from build123d import *

# Parameters (mm, degrees)
BASE_FLANGE1_START             = -11.5
BASE_FLANGE1_DEPTH             = 23
EDGE_FLANGE1_STRIP_W           = 7.0732
EDGE_FLANGE1_STRIP_H           = 1.4
EDGE_FLANGE1_STRIP_CUT_DEPTH   = 39.1268
EDGE_FLANGE1_STRIP_2_W         = 7.0732
EDGE_FLANGE1_STRIP_2_H         = 1.4
EDGE_FLANGE1_STRIP_CUT_2_DEPTH = 39.1268
EDGE_FLANGE1_DEPTH             = 39.1268
EDGE_FLANGE1_BEND_DEPTH        = 39.1268
FILLET1_RADIUS                 = 11.5
FILLET1_LENGTH                 = 1.4
CUT_EXTRUDE1_REACH             = 58.319
SKETCH12_R                     = 4.05
SKETCH12_R_2                   = 0.9
SKETCH13_R                     = 4.075
SKETCH13_R_2                   = 0.9
CUT_EXTRUDE2_DEPTH             = 42.942102952
FILLET2_R                      = 0.5
CUT_EXTRUDE3_REACH             = 58.319
SKETCH14_R                     = 4.05
SKETCH14_R_2                   = 0.9


# Read off the part's stored shape, not the designer's step: Base-Flange1
# Sheet-metal steps are written as plain solids
with BuildPart() as part:
    # Base-Flange1 outline → Base-Flange1 (new body)
    with BuildSketch(Plane(origin=(0, 0, 0), x_dir=(0, 0, -1), z_dir=(1, 0, 0)).offset(BASE_FLANGE1_START)):
        with BuildLine():
            Line((21.7, 2.1366), (21.7, 34))
            Line((21.7, 34), (20.3, 34))
            Line((20.3, 34), (20.3, 2.1366))
            ThreePointArc((20.3, 2.1366), (20.084254855, 1.615745145), (19.5634, 1.4))
            Line((19.5634, 1.4), (-19.5634, 1.4))
            ThreePointArc((-19.5634, 1.4), (-20.084254855, 1.615745145), (-20.3, 2.1366))
            Line((-20.3, 2.1366), (-20.3, 34))
            Line((-20.3, 34), (-21.7, 34))
            Line((-21.7, 34), (-21.7, 2.1366))
            ThreePointArc((-21.7, 2.1366), (-21.074204349, 0.625795651), (-19.5634, 0))
            Line((-19.5634, 0), (19.5634, 0))
            ThreePointArc((19.5634, 0), (21.074204349, 0.625795651), (21.7, 2.1366))
        make_face()
    extrude(amount=BASE_FLANGE1_DEPTH)

    # Edge-Flange1 strip (across the edge) → Edge-Flange1 strip cut (cut)
    with BuildSketch(Plane(origin=(11.5, 1.4, 19.5634), x_dir=(-1, 0, 0), z_dir=(0, 0, -1))):
        with Locations((-1.4, -0.7)):
            Rectangle(EDGE_FLANGE1_STRIP_W, EDGE_FLANGE1_STRIP_H)
    extrude(amount=EDGE_FLANGE1_STRIP_CUT_DEPTH, mode=Mode.SUBTRACT)

    # Edge-Flange1 strip 2 (across the edge) → Edge-Flange1 strip cut 2 (cut)
    with BuildSketch(Plane(origin=(-11.5, 1.4, -19.5634), x_dir=(1, 0, 0), z_dir=(0, 0, 1))):
        with Locations((-1.4, -0.7)):
            Rectangle(EDGE_FLANGE1_STRIP_2_W, EDGE_FLANGE1_STRIP_2_H)
    extrude(amount=EDGE_FLANGE1_STRIP_CUT_2_DEPTH, mode=Mode.SUBTRACT)

    # Edge-Flange1 section (across the edge) → Edge-Flange1 (add)
    with BuildSketch(Plane(origin=(11.5, 1.4, 19.5634), x_dir=(-1, 0, 0), z_dir=(0, 0, -1))):
        with BuildLine():
            Line((0, 0.7366), (0, 3.6))
            Line((0, 3.6), (1.4, 3.6))
            Line((1.4, 3.6), (1.4, 0.7366))
            ThreePointArc((1.4, 0.7366), (1.615745145, 0.215745145), (2.1366, 0))
            Line((2.1366, 0), (2.1366, -1.4))
            ThreePointArc((2.1366, -1.4), (0.625795651, -0.774204349), (0, 0.7366))
        make_face()
    extrude(amount=EDGE_FLANGE1_DEPTH)

    # Edge-Flange1 section 2 (across the edge) → Edge-Flange1 bend (add)
    with BuildSketch(Plane(origin=(-11.5, 1.4, -19.5634), x_dir=(1, 0, 0), z_dir=(0, 0, 1))):
        with BuildLine():
            Line((0, 0.7366), (0, 3.6))
            Line((0, 3.6), (1.4, 3.6))
            Line((1.4, 3.6), (1.4, 0.7366))
            ThreePointArc((1.4, 0.7366), (1.615745145, 0.215745145), (2.1366, 0))
            Line((2.1366, 0), (2.1366, -1.4))
            ThreePointArc((2.1366, -1.4), (0.625795651, -0.774204349), (0, 0.7366))
        make_face()
    extrude(amount=EDGE_FLANGE1_BEND_DEPTH)

    # Fillet1: full round fillet: the end face becomes a half cylinder, R = half its width
    fillet1_face = Plane((0, 34, 21), x_dir=(0, 0, 1), z_dir=(0, 1, 0))  # on the end face: x along it, z out of the body
    fillet1_slab = fillet1_face.offset(-FILLET1_RADIUS / 2) * Box(FILLET1_LENGTH, 2 * FILLET1_RADIUS, FILLET1_RADIUS, mode=Mode.PRIVATE)  # the body's end, R deep
    fillet1_round = Plane((0, 22.5, 21), x_dir=(0, 1, 0), z_dir=(0, 0, 1)) * Cylinder(FILLET1_RADIUS, FILLET1_LENGTH, mode=Mode.PRIVATE)  # its axis R under the face
    add(fillet1_slab - fillet1_round, mode=Mode.SUBTRACT)

    # Sketch12 → Cut-Extrude1 (cut, up to next)
    with BuildSketch(Plane.XY.offset(21.7), mode=Mode.PRIVATE) as cut_extrude1_sk1:
        with Locations((0, 22.5)):
            Circle(SKETCH12_R)
    cut_extrude1_tool1 = extrude(cut_extrude1_sk1.sketch, amount=-CUT_EXTRUDE1_REACH, mode=Mode.PRIVATE) & part.part
    # Sketch12 → Cut-Extrude1 (cut, up to next)
    with BuildSketch(Plane.XY.offset(21.7), mode=Mode.PRIVATE) as cut_extrude1_sk2:
        with Locations((0, 29.5)):
            Circle(SKETCH12_R_2)
    cut_extrude1_tool2 = extrude(cut_extrude1_sk2.sketch, amount=-CUT_EXTRUDE1_REACH, mode=Mode.PRIVATE) & part.part
    # Sketch12 → Cut-Extrude1 (cut, up to next)
    with BuildSketch(Plane.XY.offset(21.7), mode=Mode.PRIVATE) as cut_extrude1_sk3:
        with Locations((7, 22.5)):
            Circle(SKETCH12_R_2)
    cut_extrude1_tool3 = extrude(cut_extrude1_sk3.sketch, amount=-CUT_EXTRUDE1_REACH, mode=Mode.PRIVATE) & part.part
    # Sketch12 → Cut-Extrude1 (cut, up to next)
    with BuildSketch(Plane.XY.offset(21.7), mode=Mode.PRIVATE) as cut_extrude1_sk4:
        with Locations((0, 15.5)):
            Circle(SKETCH12_R_2)
    cut_extrude1_tool4 = extrude(cut_extrude1_sk4.sketch, amount=-CUT_EXTRUDE1_REACH, mode=Mode.PRIVATE) & part.part
    # Sketch12 → Cut-Extrude1 (cut, up to next)
    with BuildSketch(Plane.XY.offset(21.7), mode=Mode.PRIVATE) as cut_extrude1_sk5:
        with Locations((-7, 22.5)):
            Circle(SKETCH12_R_2)
    cut_extrude1_tool5 = extrude(cut_extrude1_sk5.sketch, amount=-CUT_EXTRUDE1_REACH, mode=Mode.PRIVATE) & part.part
    add(cut_extrude1_tool1.solids().sort_by_distance((0, 22.5, 21.7))[0], mode=Mode.SUBTRACT)
    add(cut_extrude1_tool2.solids().sort_by_distance((0, 29.5, 21.7))[0], mode=Mode.SUBTRACT)
    add(cut_extrude1_tool3.solids().sort_by_distance((7, 22.5, 21.7))[0], mode=Mode.SUBTRACT)
    add(cut_extrude1_tool4.solids().sort_by_distance((0, 15.5, 21.7))[0], mode=Mode.SUBTRACT)
    add(cut_extrude1_tool5.solids().sort_by_distance((-7, 22.5, 21.7))[0], mode=Mode.SUBTRACT)

    # Sketch13 → Cut-Extrude2 (cut, through all)
    with BuildSketch(Plane(origin=(0, 0, 0), x_dir=(1, 0, 0), z_dir=(0, 1, 0))):
        with Locations(Location((0, 0, 0), (0, 0, 270))):
            Circle(SKETCH13_R)
        with Locations(Location((-4.87903679, 4.87903679, 0), (0, 0, 270))):
            Circle(SKETCH13_R_2)
        with Locations(Location((4.87903679, 4.87903679, 0), (0, 0, 270))):
            Circle(SKETCH13_R_2)
        with Locations(Location((4.87903679, -4.87903679, 0), (0, 0, 270))):
            Circle(SKETCH13_R_2)
        with Locations(Location((-4.87903679, -4.87903679, 0), (0, 0, 270))):
            Circle(SKETCH13_R_2)
        with Locations(Location((0, 13.35, 0), (0, 0, 270))):
            Circle(SKETCH13_R_2)
        with Locations(Location((0, -13.35, 0), (0, 0, 90))):
            Circle(SKETCH13_R_2)
    extrude(amount=CUT_EXTRUDE2_DEPTH, mode=Mode.SUBTRACT)

    # Fillet2
    fillet2_edges = [part.edges().sort_by_distance(p)[0] for p in [
        (-11.5, 34, -21),
        (11.5, 34, -21),
    ]]
    fillet(fillet2_edges, radius=FILLET2_R)

    # Sketch14 → Cut-Extrude3 (cut, up to next)
    with BuildSketch(Plane(origin=(0, 0, -21.7), x_dir=(-1, 0, 0), z_dir=(0, 0, -1)), mode=Mode.PRIVATE) as cut_extrude3_sk1:
        with Locations(Location((0, 22.5, 0), (0, 0, 180))):
            Circle(SKETCH14_R)
    cut_extrude3_tool1 = extrude(cut_extrude3_sk1.sketch, amount=-CUT_EXTRUDE3_REACH, mode=Mode.PRIVATE) & part.part
    # Sketch14 → Cut-Extrude3 (cut, up to next)
    with BuildSketch(Plane(origin=(0, 0, -21.7), x_dir=(-1, 0, 0), z_dir=(0, 0, -1)), mode=Mode.PRIVATE) as cut_extrude3_sk2:
        with Locations(Location((-7.5, 30, 0), (0, 0, 90))):
            Circle(SKETCH14_R_2)
    cut_extrude3_tool2 = extrude(cut_extrude3_sk2.sketch, amount=-CUT_EXTRUDE3_REACH, mode=Mode.PRIVATE) & part.part
    # Sketch14 → Cut-Extrude3 (cut, up to next)
    with BuildSketch(Plane(origin=(0, 0, -21.7), x_dir=(-1, 0, 0), z_dir=(0, 0, -1)), mode=Mode.PRIVATE) as cut_extrude3_sk3:
        with Locations(Location((7.5, 30, 0), (0, 0, 90))):
            Circle(SKETCH14_R_2)
    cut_extrude3_tool3 = extrude(cut_extrude3_sk3.sketch, amount=-CUT_EXTRUDE3_REACH, mode=Mode.PRIVATE) & part.part
    # Sketch14 → Cut-Extrude3 (cut, up to next)
    with BuildSketch(Plane(origin=(0, 0, -21.7), x_dir=(-1, 0, 0), z_dir=(0, 0, -1)), mode=Mode.PRIVATE) as cut_extrude3_sk4:
        with Locations(Location((7.5, 15, 0), (0, 0, 90))):
            Circle(SKETCH14_R_2)
    cut_extrude3_tool4 = extrude(cut_extrude3_sk4.sketch, amount=-CUT_EXTRUDE3_REACH, mode=Mode.PRIVATE) & part.part
    # Sketch14 → Cut-Extrude3 (cut, up to next)
    with BuildSketch(Plane(origin=(0, 0, -21.7), x_dir=(-1, 0, 0), z_dir=(0, 0, -1)), mode=Mode.PRIVATE) as cut_extrude3_sk5:
        with Locations(Location((-7.5, 15, 0), (0, 0, 90))):
            Circle(SKETCH14_R_2)
    cut_extrude3_tool5 = extrude(cut_extrude3_sk5.sketch, amount=-CUT_EXTRUDE3_REACH, mode=Mode.PRIVATE) & part.part
    add(cut_extrude3_tool1.solids().sort_by_distance((0, 22.5, -21.7))[0], mode=Mode.SUBTRACT)
    add(cut_extrude3_tool2.solids().sort_by_distance((7.5, 30, -21.7))[0], mode=Mode.SUBTRACT)
    add(cut_extrude3_tool3.solids().sort_by_distance((-7.5, 30, -21.7))[0], mode=Mode.SUBTRACT)
    add(cut_extrude3_tool4.solids().sort_by_distance((-7.5, 15, -21.7))[0], mode=Mode.SUBTRACT)
    add(cut_extrude3_tool5.solids().sort_by_distance((7.5, 15, -21.7))[0], mode=Mode.SUBTRACT)


solid = part.part
Input: part model. Units: mm. Frame: model coordinates. A direction names the side the tool comes from. Coordinates: 2 decimals unless noted, no trailing zeros. Loops run counter-clockwise (first coordinate to the right, second up) from the corner with the lowest first, then second, coordinate; pieces in that order, holes last.
(1) Section D-D on z = -8. Return the cut outline in (x, y), then the cut area to 3 significant figures.
(2) Section C-C on x = 3.25. Return the cut outline in (y, z), then the cut area to 3 significant figures.
(3) Material intervals for probe 1 along Y at (x, z) = (0, 21.3); probe 2 along X at (y, z) = (15, -21); probe 3 along Z at (x, y) = (8.75, 10.5), sorted ascending.
(4) Section A-A on y = 3. Return the cut outline in (x, z), then the cut area to 3 significant figures.
(5) Pull-direction query (X, two-part tool) for faces 5 (the face through (-11.5, 11, 21)), 6 (the face through (4.92, 0.69, 3.98)), 7 (the face through (-11, 0.4, -19.563)); classes: released by +X, released by -X, zero draft, split by the parting line, or undercut.
(6) First-contact query: pin 1 Ø2.5 at (x, z) = (-4.88, -4.88) entering from +Y; pin 2 Ø10.5 at (x, z) = (0, 0) entering from -Y; pin 3 Ø0.7 at (x, z) = (-11, 6) entering from +Y; pin 4 Ø10 at (y, z) = (18.5, 12) entering from -X. Flat tips, straight axial feed; report the tip coordinate or a pass-through.
(7) Set-up query: faces 1 (the face through (-11, 0.4, 19.563)), 2 (the face through (-4.3, 1.4, -0.3)), 3 (the face through (-7.12, 23.39, 21.01)), 4 (the face through (11, 0.4, 19.563)). Return all of +Z, -Z, +X, -X, +Y, -Y with unobstructed straight access to the full face (end or side cutting, diameter ignored); none if empty.
(8) Section B-B on z = 13.35. Return the cut outline in (x, y).
Data:
1. outline: (-11.5, 2.14) arc R2.14 ccw to (-9.36, 0) - (9.36, 0) arc R2.14 ccw to (11.5, 2.14) - (11.5, 5) - (10.1, 5) - (10.1, 2.14) arc R0.74 cw to (9.36, 1.4) - (-9.36, 1.4) arc R0.74 cw to (-10.1, 2.14) - (-10.1, 5) - (-11.5, 5) - close
1. area: 40.6 mm2
2. outline: (0, -19.56) arc R2.14 ccw to (2.14, -21.7) - (20.08, -21.7) - (20.08, -20.3) - (2.14, -20.3) arc R0.74 cw to (1.4, -19.56) - (1.4, -2.46) - (0, -2.46) - close; (0, 2.46) - (1.4, 2.46) - (1.4, 19.56) arc R0.74 cw to (2.14, 20.3) - (20.08, 20.3) - (20.08, 21.7) - (2.14, 21.7) arc R2.14 ccw to (0, 19.56) - close; (24.92, -21.7) - (34, -21.7) - (34, -20.3) - (24.92, -20.3) - close; (24.92, 20.3) - (33.53, 20.3) - (33.53, 21.7) - (24.92, 21.7) - close
2. area: 129 mm2
3. probe 1: y = 0.89 to 14.6, 16.4 to 18.45, 26.55 to 28.6, 30.4 to 34
3. probe 2: x = -11.5 to -8.4, -6.6 to 6.6, 8.4 to 11.5
3. probe 3: z = -21.7 to -20.3, 20.3 to 21.7
4. outline: (-11.5, -21.7) - (11.5, -21.7) - (11.5, -20.3) - (-11.5, -20.3) - close; (-11.5, -19.56) - (-10.1, -19.56) - (-10.1, 19.56) - (-11.5, 19.56) - close; (-11.5, 20.3) - (11.5, 20.3) - (11.5, 21.7) - (-11.5, 21.7) - close; (10.1, -19.56) - (11.5, -19.56) - (11.5, 19.56) - (10.1, 19.56) - close
4. area: 174 mm2
5. face 5: released by -X
5. face 6: undercut
5. face 7: zero draft
6. pin 1: stops at y = 1.4
6. pin 2: stops at y = 0
6. pin 3: stops at y = 5
6. pin 4: passes through
7. face 1: -X, -Y
7. face 2: +Y
7. face 3: +Z
7. face 4: +X, -Y
8. outline: (-11.5, 2.14) arc R2.14 ccw to (-9.36, 0) - (-0.9, 0) - (-0.9, 1.4) - (-9.36, 1.4) arc R0.74 cw to (-10.1, 2.14) - (-10.1, 5) - (-11.5, 5) - close; (0.9, 0) - (9.36, 0) arc R2.14 ccw to (11.5, 2.14) - (11.5, 5) - (10.1, 5) - (10.1, 2.14) arc R0.74 cw to (9.36, 1.4) - (0.9, 1.4) - close
